For this review, use the dimensioned drawing (mm, ordinates from the lowest corner) and the shaded views. A direction names the side the tool comes from. Coordinates: 2 decimals unless noted, no trailing zeros. Write each loop counter-clockwise with the first axis right and the second up, starting at its lowest first coordinate (ties: lowest second). Pieces come first, ordered by that corner, then holes. Notation, with made-up numbers: (23, 51) - (59, 51) arc R16 cw to (59, 62) - close; hole circle Ø4 at (39, 26.5). An arc over 180 degrees is marked (long way). Use one line per item in the form item = value. Start each with the question number.
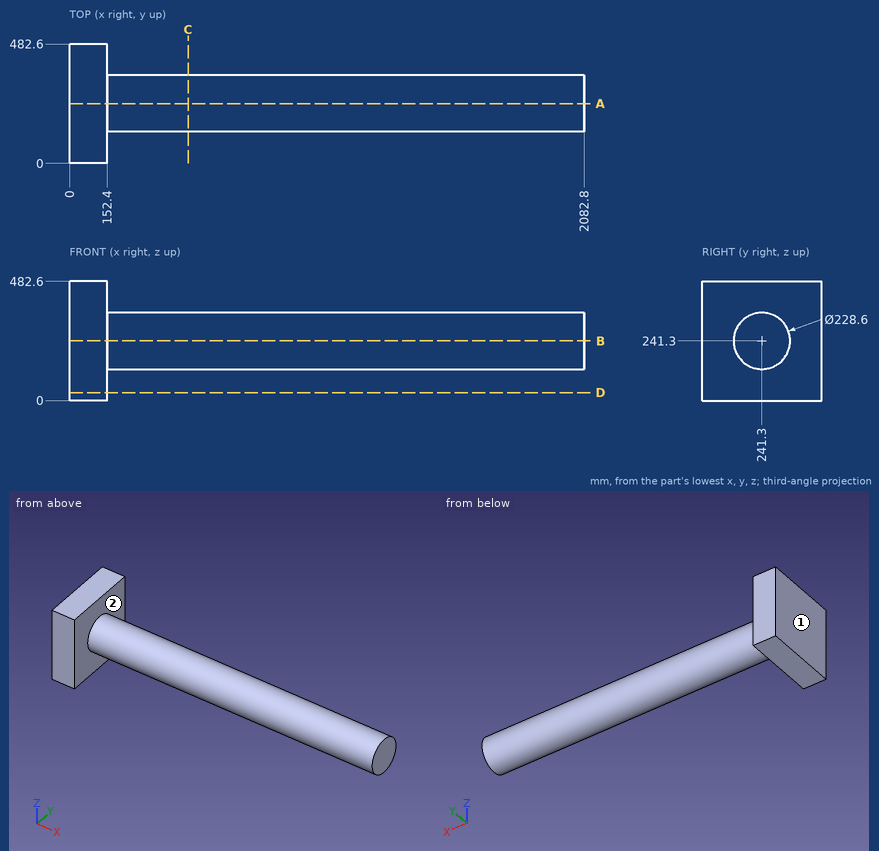
1. Take a section at C-C (x = 479.5). State the section outline as (y, z) points.
2. For P1, Ø1.5, axis at x = 281.5, z = 160, coming from the -Y side; P2, Ø5, axis at y = 267.5, z = 381, coming from the +X side; P3, Ø12, axis at x = 1366, y = 353, coming from the +Z side, all flat-tipped, find the tip position at first contact; note any pin that passes through.
3. Take a section at A-A (y = 241.3). State the section outline as (x, z) points, plus the area to 3 significant figures.
4. For L1, parallel to X at y = 195.5, z = 84.5; L2, parallel to Z at x = 225, y = 251; L3, parallel to Y at x = 1465, z = 249, list the stretches that pass through material, from the lowest coordinate up.
5. For the marked faces 1 and 2, list the 3-axis set-ups (+Z, -Z, +X, -X, +Y, -Y) from which the entire face can be reached by the end or side of a thin tool; tool diameter is ignored.
6. Take a section at D-D (z = 31.5). State the section outline as (x, y) points.
Returned:
q1.outline = circle Ø228.6 at (241.3, 241.3)
q2.P1 = 160.21
q2.P2 = 152.4
q2.P3 = 284.8
q3.outline = (0, 0) - (152.4, 0) - (152.4, 127) - (2082.8, 127) - (2082.8, 355.6) - (152.4, 355.6) - (152.4, 482.6) - (0, 482.6) - close
q3.area = 515,000 mm²
q4.L1 = 0 to 152.4
q4.L2 = 127.41 to 355.19
q4.L3 = 127.26 to 355.34
q5.face_1 = +Z, -Z, -X, +Y, -Y
q5.face_2 = +X
q6.outline = (0, 0) - (152.4, 0) - (152.4, 482.6) - (0, 482.6) - close
